from build123d import *

# Parameters (mm, degrees)
SKETCH_1_W          = 100.539230484
SKETCH_1_H          = 40
SKETCH_1_W_2        = 17
SKETCH_1_H_2        = 7
EXTRUDE_1_DEPTH     = 2
SKETCH_2_W          = 100.539230484
SKETCH_2_H          = 40
SKETCH_2_R          = 2.25
EXTRUDE_2_DEPTH     = 1.5
SKETCH_3_W          = 184.808915215
SKETCH_3_H          = 94.825170589
CUT_EXTRUDE_1_DEPTH = 31.5


with BuildPart() as part:
    # Sketch 1 → Extrude 1 (new body)
    with BuildSketch(Plane.XY):
        with Locations((62.5, 12.5)):
            Rectangle(SKETCH_1_W, SKETCH_1_H)
        with Locations((24.230384758, 25)):
            Rectangle(SKETCH_1_W_2, SKETCH_1_H_2, mode=Mode.SUBTRACT)
        with Locations((100.769615242, 0)):
            Rectangle(SKETCH_1_W_2, SKETCH_1_H_2, mode=Mode.SUBTRACT)
    extrude(amount=EXTRUDE_1_DEPTH)

    # Sketch 2 → Extrude 2 (add)
    with BuildSketch(Plane.XY.offset(2)):
        with Locations((62.5, 12.5)):
            Rectangle(SKETCH_2_W, SKETCH_2_H)
        with Locations((21.230384758, 25)):
            Circle(SKETCH_2_R, mode=Mode.SUBTRACT)
        with Locations((103.769615242, 0)):
            Circle(SKETCH_2_R, mode=Mode.SUBTRACT)
    extrude(amount=EXTRUDE_2_DEPTH)

    # Sketch 3 → Cut-Extrude 1 (cut)
    with BuildSketch(Plane.XY.offset(3.5)):
        with Locations((81.231416835, 7.831688581)):
            Rectangle(SKETCH_3_W, SKETCH_3_H)
        Polygon((12.230384758, 32.5), (42.230384758, 32.5), (54.020384758, 20.71), (75.769615242, 20.71), (88.979615242, 7.5), (112.769615242, 7.5), (112.769615242, -7.5), (82.769615242, -7.5), (66.982818678, 8.286796564), (45.230384758, 8.286796564), (36.017181322, 17.5), (12.230384758, 17.5), align=None, mode=Mode.SUBTRACT)
    extrude(amount=-CUT_EXTRUDE_1_DEPTH, mode=Mode.SUBTRACT)


solid = part.part
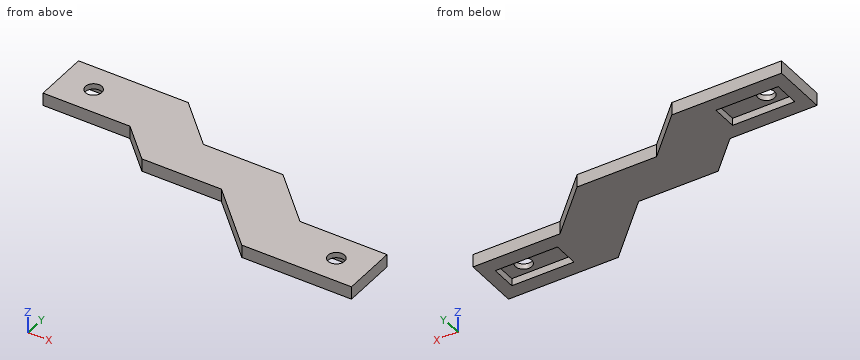
The listing builds one solid part. Answer for the finished solid, in the listing's coordinates (mm). Round coordinates to 2 decimals unless told otherwise and drop trailing zeros. Write each loop counter-clockwise with the first axis right and the second up, starting at its lowest first coordinate (ties: lowest second). Pieces come first, ordered by that corner, then holes. Notation, with made-up numbers: M 50,-28 L 55,-28 A20 ccw 55,-18 Z; hole C 45,6 d4. An arc over 180 degrees is marked long. Write each question's results on one line, items separated by ' | '. Start each with the question number.
Item 1: A cutting plane is placed at D-D on x = 64.5. Write down the section's boundary in (y, z), and give its area (3 significant figures).
Item 2: Straight lines are drawn through the part: L1, parallel to Y at x = 62, z = 2.95; L2, parallel to X at y = -2, z = 2.7; L3, parallel to X at y = -0.5, z = 2.6. For each, find the intervals that lie inside material, in ascending order. Write a range as [from, to].
Item 3: Flat-ended cylindrical pins translate along their axes: pin 1 Ø1 at (x, z) = (66, 1) entering from +Y; pin 2 Ø1.8 at (x, z) = (98, 2) entering from +Y; pin 3 Ø1 at (y, z) = (-2, 2.5) entering from -X. Find the tip coordinate at first contact, or state that the pin passes through.
Item 4: A cutting plane is placed at B-B on y = 25. Write down the section's boundary in (x, z).
Item 5: A cutting plane is placed at A-A on x = 20. Write down the section's boundary in (y, z), and give its area (3 significant figures).
Item 6: A cutting plane is placed at C-C on z = 1.25. Write down the section's boundary in (x, y).
Check sheet entries:
1) outline: M 8.29,0 L 20.71,0 L 20.71,3.5 L 8.29,3.5 Z | area: 43.5 mm²
2) L1: [8.29, 20.71] | L2: [77.27, 102.74], [104.8, 112.77] | L3: [75.77, 101.58], [105.96, 112.77]
3) pin 1: y = 20.71 | pin 2: y = 7.5 | pin 3: x = 76.77
4) outline: M 12.23,0 L 15.73,0 L 15.73,2 L 18.98,2 L 18.98,3.5 L 12.23,3.5 Z; M 23.48,2 L 32.73,2 L 32.73,0 L 49.73,0 L 49.73,3.5 L 23.48,3.5 Z
5) outline: M 17.5,0 L 21.5,0 L 21.5,2 L 23.12,2 L 23.12,3.5 L 17.5,3.5 Z; M 26.88,2 L 28.5,2 L 28.5,0 L 32.5,0 L 32.5,3.5 L 26.88,3.5 Z | area: 32.8 mm²
6) outline: M 12.23,17.5 L 36.02,17.5 L 45.23,8.29 L 66.98,8.29 L 82.77,-7.5 L 112.77,-7.5 L 112.77,7.5 L 88.98,7.5 L 75.77,20.71 L 54.02,20.71 L 42.23,32.5 L 12.23,32.5 Z; hole M 15.73,21.5 L 32.73,21.5 L 32.73,28.5 L 15.73,28.5 Z; hole M 92.27,-3.5 L 109.27,-3.5 L 109.27,3.5 L 92.27,3.5 Z
